Could you check a few things on this model? Use its own coordinates, in mm. Round coordinates to 2 decimals unless told otherwise and drop trailing zeros. Write each loop counter-clockwise with the first axis right and the second up, starting at its lowest first coordinate (ties: lowest second). Pieces come first, ordered by that corner, then holes.
Autodesk Inventor part; units mm, degrees
ref_plane "YZ Plane" through (0, 0, 0) normal (1, 0, 0) x (0, 1, 0)
ref_plane "XZ Plane" through (0, 0, 0) normal (0, 1, 0) x (-1, 0, 0)
ref_plane "XY Plane" through (0, 0, 0) normal (0, 0, 1) x (1, 0, 0)
sketch "Sketch1" plane through (0, 0, 0) normal (0, 1, 0) x (-1, 0, 0)
  line L0 (15.892, 0.4112) -> (15.892, -0.4526)
  line L1 (15.392, -0.9526) -> (11.943, -0.9526)
  line L2 (11.943, 0.9112) -> (15.392, 0.9112)
  line L3 (15.392, 0.9112) -> (11.943, 0.9112)
  line L4 (15.892, -0.4526) -> (15.892, 0.4112)
  line L5 (15.392, -0.9526) -> (11.943, -0.9526)
  line L6 (11.943, -0.9526) -> (15.392, -0.9526)
  line L7 (-39.4963, 2.5258) -> (-39.4963, 1.1377)
  line L8 (-39.4963, -1.0763) -> (-39.4963, -2.4644)
  line L9 (-42.6438, 0.6377) -> (-41.2386, 0.6377)
  line L10 (-38.9963, 0.6377) -> (-37.5911, 0.6377)
  line L11 (-40.7386, -2.4644) -> (-40.7386, -1.0763)
  line L12 (-40.7386, 1.1377) -> (-40.7386, 2.5258)
  line L13 (-37.5911, -0.5763) -> (-38.9963, -0.5763)
  line L14 (-41.2386, -0.5763) -> (-42.6438, -0.5763)
  line L15 (-37.0911, 0.1377) -> (-37.0911, -0.0763)
  line L16 (-39.9963, -2.9644) -> (-40.2386, -2.9644)
  line L17 (-43.1438, -0.0763) -> (-43.1438, 0.1377)
  line L18 (-40.2386, 3.0258) -> (-39.9963, 3.0258)
  arc A0 (-39.4963, 2.5258) -> (-39.9963, 3.0258) centre (-39.9963, 2.5258) ccw
  arc A1 (-40.2386, 3.0258) -> (-40.7386, 2.5258) centre (-40.2386, 2.5258) ccw
  arc A2 (-41.2386, 0.6377) -> (-40.7386, 1.1377) centre (-41.2386, 1.1377) ccw
  arc A3 (-42.6438, 0.6377) -> (-43.1438, 0.1377) centre (-42.6438, 0.1377) ccw
  arc A4 (-43.1438, -0.0763) -> (-42.6438, -0.5763) centre (-42.6438, -0.0763) ccw
  arc A5 (-40.7386, -1.0763) -> (-41.2386, -0.5763) centre (-41.2386, -1.0763) ccw
  arc A6 (-40.7386, -2.4644) -> (-40.2386, -2.9644) centre (-40.2386, -2.4644) ccw
  arc A7 (-39.9963, -2.9644) -> (-39.4963, -2.4644) centre (-39.9963, -2.4644) ccw
  arc A8 (-38.9963, -0.5763) -> (-39.4963, -1.0763) centre (-38.9963, -1.0763) ccw
  arc A9 (-39.4963, 1.1377) -> (-38.9963, 0.6377) centre (-38.9963, 1.1377) ccw
  arc A10 (-37.0911, 0.1377) -> (-37.5911, 0.6377) centre (-37.5911, 0.1377) ccw
  arc A11 (-37.5911, -0.5763) -> (-37.0911, -0.0763) centre (-37.5911, -0.0763) ccw
  line L19 (-45, 8) -> (-45, -8)
  line L20 (11.443, 0.4112) -> (11.443, -0.4526)
  arc A12 (15.392, -0.9526) -> (15.892, -0.4526) centre (15.392, -0.4526) ccw
  arc A13 (15.892, 0.4112) -> (15.392, 0.9112) centre (15.392, 0.4112) ccw
  arc A14 (11.943, 0.9112) -> (11.443, 0.4112) centre (11.943, 0.4112) ccw
  arc A15 (11.443, -0.4526) -> (11.943, -0.9526) centre (11.943, -0.4526) ccw
  arc A16 (-43, 10) -> (-45, 8) centre (-43, 8) ccw
  arc A17 (-45, -8) -> (-43, -10) centre (-43, -8) ccw
  line L21 (-29.25, -2) -> (-29.25, 2) construction
  line L22 (-15, -10) -> (11, -10)
  line L23 (15.5, -10) -> (18, -10)
  line L24 (18, 10) -> (15.5, 10)
  line L25 (11, 10) -> (-30, 10)
  line L26 (-15, -10) -> (10, -10)
  line L27 (-12.5, 7) -> (-12.5, 30.9822) construction
  line L28 (-12.5, -7) -> (-12.5, -36.1495) construction
  line L29 (-30, 10) -> (-36, 10)
  line L30 (-40.5, 10) -> (-43, 10)
  line L31 (-43, -10) -> (-40.5, -10)
  line L32 (-36, -10) -> (-15, -10)
  line L33 (-43.1438, 0) -> (-43.1438, -0.0763) construction
  line L34 (-43, -10) -> (-43, -10) construction
  line L35 (20, -8) -> (20, 8)
  arc A18 (18, -10) -> (20, -8) centre (18, -8) ccw
  arc A19 (20, 8) -> (18, 10) centre (18, 8) ccw
  line L36 (15.5, -10) -> (18, -10)
  line L37 (18, 10) -> (15.5, 10)
  line L38 (15.5, -10) -> (15.5, -11.75)
  line L39 (15.25, -12) -> (11.25, -12)
  line L40 (11, -11.75) -> (11, -10)
  line L41 (15.5, 10) -> (15.5, 11.75)
  line L42 (11, 11.75) -> (11, 10)
  line L43 (-36, 10) -> (-36, 11.75)
  line L44 (-36.25, 12) -> (-40.25, 12)
  line L45 (-40.5, 11.75) -> (-40.5, 10)
  line L46 (-36, -10) -> (-36, -11.75)
  line L47 (-36.25, -12) -> (-40.25, -12)
  line L48 (-40.5, -10) -> (-40.5, -11.75)
  arc A20 (-36, 11.75) -> (-36.25, 12) centre (-36.25, 11.75) ccw
  arc A21 (-40.25, 12) -> (-40.5, 11.75) centre (-40.25, 11.75) ccw
  arc A22 (-40.5, -11.75) -> (-40.25, -12) centre (-40.25, -11.75) ccw
  arc A23 (-36.25, -12) -> (-36, -11.75) centre (-36.25, -11.75) ccw
  arc A24 (15.25, -12) -> (15.5, -11.75) centre (15.25, -11.75) ccw
  arc A25 (11, -11.75) -> (11.25, -12) centre (11.25, -11.75) ccw
  arc A26 (15.5, 11.75) -> (15.25, 12) centre (15.25, 11.75) ccw
  arc A27 (11.25, 12) -> (11, 11.75) centre (11.25, 11.75) ccw
  line L49 (11.25, 12) -> (15.25, 12)
  line L50 (-29.25, 0) -> (-14.25, 0) construction
  line L51 (-29.25, 0) -> (-14.25, 0) construction
  line L52 (-29.25, -4) -> (-14.25, -4)
  line L53 (-14.25, 4) -> (-29.25, 4)
  arc A28 (-14.25, -4) -> (-14.25, 4) centre (-14.25, 0) ccw
  line L54 (-32.6715, -2.0721) -> (-33.7507, -0.2901)
  line L55 (-33.7546, 0.2214) -> (-32.7027, 2.0197)
  arc A29 (-29.25, 4) -> (-32.7027, 2.0197) centre (-29.25, 0) ccw
  arc A30 (-32.6715, -2.0721) -> (-29.25, -4) centre (-29.25, 0) ccw
  arc A31 (-33.7546, 0.2214) -> (-33.7507, -0.2901) centre (-33.323, -0.0311) ccw
  point P0 (15.5, -12)
  point P1 (15.5, 12)
  point P2 (11, 12)
  point P3 (-36, 12)
  point P4 (-40.5, 12)
  point P5 (-36, -12)
  point P6 (-40.5, -12)
  point P7 (-21.75, 0)
  dimension "d2" = 0.5
  dimension "d4" = 0.5
  dimension "d38" = 2
  dimension "d40" = 0.25
  dimension "d41" = 47
  dimension "d42" = 47
  dimension "d43" = 56
  dimension "d44" = 15
  dimension "d45" = 15.75
  dimension "d46" = 8
  dimension "d47" = 0.5
extrude "Extrusion1" add sketch "Sketch1" along normal blind 2
properties part number "Laser-Slot-Bottom" material "Acrylic, Clear"
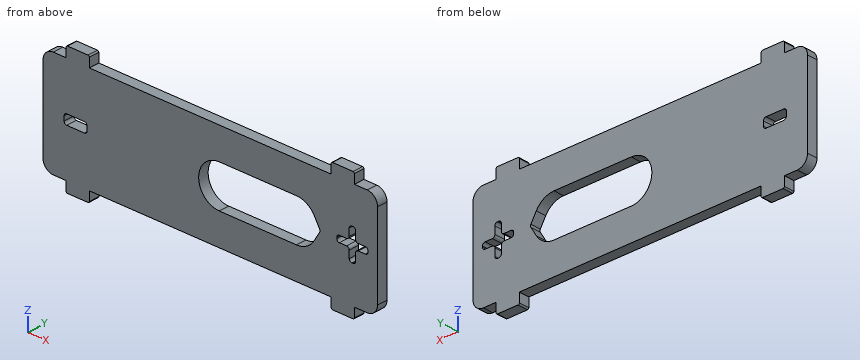
Q1. If I drill on L1, parallel to X at y = 0.9, z = -2.75; L2, parallel to Z at x = 17, y = 0.7; L3, parallel to X at y = 1.85, z = 1.5, over which ranges is the centre line in solid material (lowest first)?
Q2. Imagine slicing it at B-B, the plane x = 3. Write out the boundary of the cut face in (y, z).
Q3. Imagine slicing it at A-A, the plane y = 1.3. Count the separate pieces of the cut face and the enclosed holes in it, then the cut area to 3 significant figures.
Q4. I'm going to push flat-ended pins straight in: pin 1 Ø1 at (x, y) = (22, 1) entering from -Z; pin 2 Ø0.5 at (y, z) = (0.5, 10.5) entering from -X. Where does each tip first touch, or does it pass through?
Results found:
1. L1: x = -20 to 11.35, 32.15 to 39.59, 40.65 to 45
1. L2: z = -10 to -4, 4 to 10
1. L3: x = -20 to 10.54, 33.01 to 39.5, 40.74 to 45
2. outline: (0, -10) - (2, -10) - (2, 10) - (0, 10) - close
3. separate pieces: 1
3. enclosed holes: 3
3. area: 1,140 mm2
4. pin 1: stops at z = -10
4. pin 2: stops at x = -15.5
